CAD build for the part. Positions are in the model's coordinates, mm. A direction names the side the tool comes from. Coordinates: 2 decimals unless noted, no trailing zeros. Loops run counter-clockwise (first coordinate to the right, second up) from the corner with the lowest first, then second, coordinate; pieces in that order, holes last.
1) Saw through at D-D, the plane z = 3. Write the cut outline in (x, y).
2) Which spindle directions (+Z, -Z, +X, -X, +Y, -Y) get a long thin tool onto all of the face, cutting with end or side? Do faces 5 (the flat face through (-23, -8, 2)), 6 (the flat face through (42, -11, 8)), 7 (the cylindrical face through (39.65, -12.97, 6.94)), 8 (the flat face through (22, -8, 9)). Say none if no direction does.
3) Two-plate mould, pull along Z, no slides. Class faces 1 (the flat face through (44, -8, 9)), 2 (the flat face through (-1, -1, 0)), 3 (the flat face through (7, -11, 8)), 4 (the flat face through (22, -12, 13)): +Z half, -Z half, draft (parallel to the pull), parting line (faces both ways), or undercut.
4) Saw through at A-A, the plane z = 8.5. Write the cut outline in (x, y), and give its area (3 significant figures).
5) Saw through at B-B, the plane y = 0. Write the cut outline in (x, z).
6) Wall check: line 1 along X through (y, z) = (-9.4, 8.5); line 2 along X through (y, z) = (-13.05, 8.5); line 3 along Z through (x, y) = (40, -10.2). Give the ranges that are in metal, low to high.
7) Pin check, flat tips, straight feed: pin 1 Ø12 at (x, y) = (-17, -10.5) entering from +Z; pin 2 Ø2 at (y, z) = (-11, 4) entering from -X; pin 3 Ø1 at (x, z) = (2, 9) entering from +Y. Stop position of each tip, or through.
8) Saw through at C-C, the plane x = -37.5. Write the cut outline in (y, z), and give its area (3 significant figures).
```python
from build123d import *

# Parameters (mm, degrees)
ESBO_O1_W                  = 90
ESBO_O1_H                  = 16
ESBO_O1_R                  = 2.1
RESSALTO_EXTRUS_O1_DEPTH   = 4
ESBO_O2_W                  = 45
ESBO_O2_H                  = 13
ESBO_O2_R                  = 1.6
RESSALTO_EXTRUS_O3_DEPTH   = 7
FILETE1_R                  = 6
FILETE2_R                  = 2
CORTE_EXTRUS_O1_DEPTH      = 10
CORTE_EXTRUS_O1_DEPTH_BACK = 3
ESBO_O3_R                  = 3.1
FILETE3_R                  = 2


with BuildPart() as part:
    # Esboço1 → Ressalto-extrusão1 (new body)
    with BuildSketch(Plane.XY):
        Rectangle(ESBO_O1_W, ESBO_O1_H)
        with Locations((-37.5, 0)):
            Circle(ESBO_O1_R, mode=Mode.SUBTRACT)
        with Locations((37.5, 0)):
            Circle(ESBO_O1_R, mode=Mode.SUBTRACT)
    extrude(amount=RESSALTO_EXTRUS_O1_DEPTH)

    # Esboço2 → Ressalto-extrusão3 (add)
    with BuildSketch(Plane.XZ.offset(8)):
        with Locations((22.5, 6.5)):
            Rectangle(ESBO_O2_W, ESBO_O2_H)
        with Locations((40, 8.5)):
            Circle(ESBO_O2_R, mode=Mode.SUBTRACT)
        with Locations((5, 8.5)):
            Circle(ESBO_O2_R, mode=Mode.SUBTRACT)
    extrude(amount=RESSALTO_EXTRUS_O3_DEPTH)

    # Filete1
    filete1_edges = [part.edges().sort_by_distance(p)[0] for p in [
        (0, -8, 2),
        (-45, 8, 2),
        (45, 8, 2),
        (-45, -8, 2),
    ]]
    fillet(filete1_edges, radius=FILETE1_R)

    # Filete2
    filete2_edges = [part.edges().sort_by_distance(p)[0] for p in [
        (22.5, -8, 4),
        (0, -11, 4),
    ]]
    fillet(filete2_edges, radius=FILETE2_R)

    # Esboço3 → Corte-extrusão1 (cut, two sides: drawn at the far end of the back side and taken through both)
    with BuildSketch(Plane(origin=(0, -8, 0), x_dir=(1, 0, 0), z_dir=(0, 1, 0)).offset(-CORTE_EXTRUS_O1_DEPTH_BACK)):
        with Locations(Location((5, -8.5, 0), (0, 0, 53.750679117))):
            Circle(ESBO_O3_R)
        with Locations(Location((40, -8.5, 0), (0, 0, 53.750679117))):
            Circle(ESBO_O3_R)
    extrude(amount=CORTE_EXTRUS_O1_DEPTH + CORTE_EXTRUS_O1_DEPTH_BACK, mode=Mode.SUBTRACT)

    # Filete3
    # the kernel refuses this fillet: 2 mm, written as the material it takes off along each edge
    with BuildSketch(Plane(origin=(50, -8, 13), x_dir=(0, 0, -1), z_dir=(-1, 0, 0))) as filete3_piece_1:
        with BuildLine():
            CenterArc((FILETE3_R, FILETE3_R), FILETE3_R, 180, 90)
            Line((0, FILETE3_R), (0, 0))
            Line((0, 0), (FILETE3_R, 0))
        make_face()
    extrude(amount=55, mode=Mode.SUBTRACT)


solid = part.part
```
Data:
1. outline: (-45, -2) arc R6 ccw to (-39, -8) - (-6, -8) arc R6 cw to (0, -14) - (0, -15) - (45, -15) - (45, 2) arc R6 ccw to (39, 8) - (-39, 8) arc R6 ccw to (-45, 2) - close; hole circle Ø4.2 at (-37.5, 0); hole circle Ø4.2 at (37.5, 0)
2. face 5: +Z, -Z, -X, -Y
2. face 6: +Y
2. face 7: +Y, -Y
2. face 8: +Z, +X, -X, +Y
3. face 1: draft
3. face 2: -Z half
3. face 3: undercut
3. face 4: +Z half
4. outline: (0, -15) - (3.4, -15) - (3.4, -11) - (1.9, -11) - (1.9, -8) - (0, -8) - close; (6.6, -15) - (38.4, -15) - (38.4, -11) - (36.9, -11) - (36.9, -8) - (8.1, -8) - (8.1, -11) - (6.6, -11) - close; (41.6, -15) - (45, -15) - (45, -8) - (43.1, -8) - (43.1, -11) - (41.6, -11) - close
4. area: 252 mm2
5. outline: (-45, 0) - (-39.6, 0) - (-39.6, 4) - (-45, 4) - close; (-35.4, 0) - (35.4, 0) - (35.4, 4) - (-35.4, 4) - close; (39.6, 0) - (45, 0) - (45, 4) - (39.6, 4) - close
6. line 1: x = 0 to 1.9, 8.1 to 36.9, 43.1 to 45
6. line 2: x = 0 to 3.4, 6.6 to 38.4, 41.6 to 45
6. line 3: z = 0 to 5.4, 11.6 to 13
7. pin 1: stops at z = 4
7. pin 2: stops at x = -1.53
7. pin 3: stops at y = -8
8. outline: (-8, 0) - (-2.1, 0) - (-2.1, 4) - (-8, 4) - close; (2.1, 0) - (8, 0) - (8, 4) - (2.1, 4) - close
8. area: 47.2 mm2
